For this review, use the dimensioned drawing (mm, ordinates from the lowest corner) and the shaded views. A direction names the side the tool comes from. Coordinates: 2 decimals unless noted, no trailing zeros. Loops run counter-clockwise (first coordinate to the right, second up) from the corner with the lowest first, then second, coordinate; pieces in that order, holes last. Notation, with made-up numbers: (23, 86) - (66, 86) arc R21 ccw to (66, 101) - close; hole circle Ø11 at (73, 13). An arc over 180 degrees is marked (long way). Answer in a Markdown table with one row per item. Add a question column.
(1) We need section D-D, the plane x = 14. Write out the cut boundary in (y, z), plus the area to 3 significant figures.
(2) The part is to be moulded in two halves that separate along X. For the marked faces 4, 5, 6 and 7, say which applies: released by +X, released by -X, zero draft, split by the parting line, or undercut.
(3) To check wall thickness, follow L1, parallel to Y at x = 72.3, z = 0.8; L2, parallel to X at y = 2.5, z = 1.25; L3, parallel to X at y = 50.7, z = 1.05. State the ranges of each line that lie inside material, in increasing order. Write a range as [from, to].
(4) We need section B-B, the plane z = 3.75. Write out the cut boundary in (x, y).
(5) We need section A-A, the plane y = 50.7. Write out the cut boundary in (x, z), plus the area to 3 significant figures.
(6) We need section C-C, the plane x = 72.3. Write out the cut boundary in (y, z).
(7) Clearance check with flat-ended pins moving along their axes: pin 1 (2 mm diameter, centred on x = 49.5, y = 18.5, fed in from +Z); pin 2 (7 mm diameter, centred on x = 26, y = 6.5, fed in from +Z); pin 3 (2.5 mm diameter, centred on y = 4, z = 8, fed in from -X). State where each tip first meets the part, or that it passes through.
(8) For the marked faces 1, 2 and 3, list the 3-axis set-ups (+Z, -Z, +X, -X, +Y, -Y) from which the entire face can be reached by the end or side of a thin tool; tool diameter is ignored.
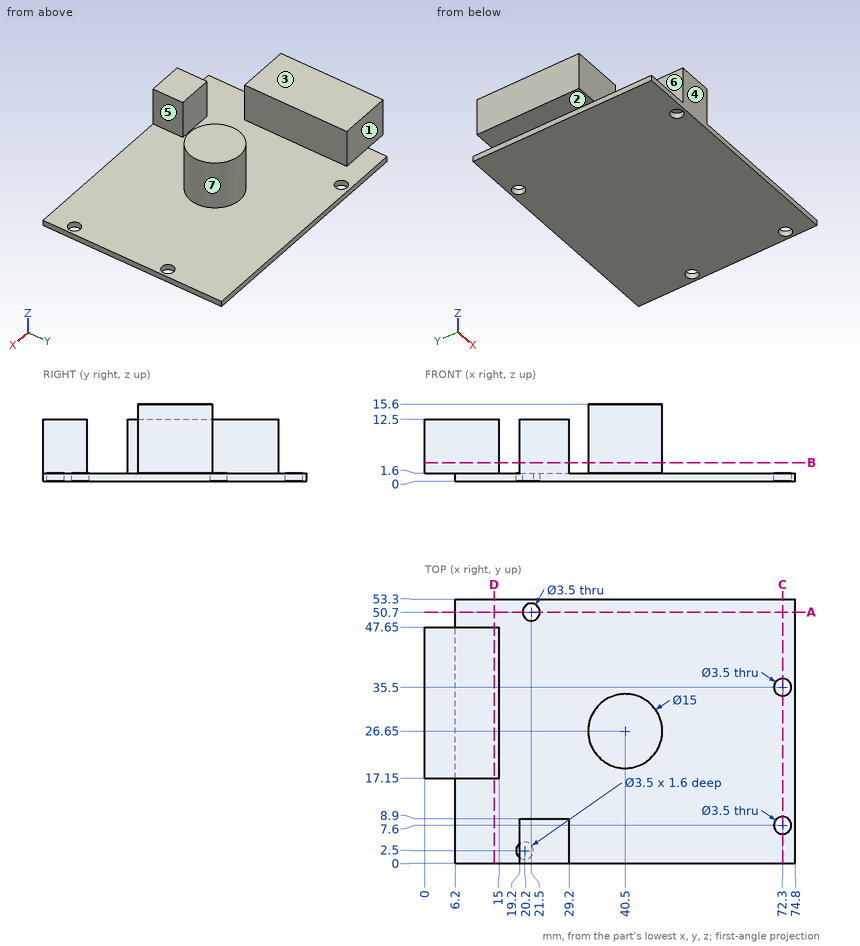
Responses:
| question | item | result |
|---|---|---|
| 1 | outline | (0, 0) - (53.3, 0) - (53.3, 1.6) - (47.65, 1.6) - (47.65, 12.5) - (17.15, 12.5) - (17.15, 1.6) - (0, 1.6) - close |
| 1 | area | 418 mm2 |
| 2 | face 4 | zero draft |
| 2 | face 5 | released by +X |
| 2 | face 6 | released by -X |
| 2 | face 7 | undercut |
| 3 | L1 | y = [0, 5.85], [9.35, 33.75], [37.25, 53.3] |
| 3 | L2 | x = [6.2, 18.45], [21.95, 74.8] |
| 3 | L3 | x = [6.2, 19.75], [23.25, 74.8] |
| 4 | outline | (0, 17.15) - (15, 17.15) - (15, 47.65) - (0, 47.65) - close; (19.2, 0) - (29.2, 0) - (29.2, 8.9) - (19.2, 8.9) - close; circle Ø15 at (40.5, 26.65) |
| 5 | outline | (6.2, 0) - (19.75, 0) - (19.75, 1.6) - (6.2, 1.6) - close; (23.25, 0) - (74.8, 0) - (74.8, 1.6) - (23.25, 1.6) - close |
| 5 | area | 104 mm2 |
| 6 | outline | (0, 0) - (5.85, 0) - (5.85, 1.6) - (0, 1.6) - close; (9.35, 0) - (33.75, 0) - (33.75, 1.6) - (9.35, 1.6) - close; (37.25, 0) - (53.3, 0) - (53.3, 1.6) - (37.25, 1.6) - close |
| 7 | pin 1 | stops at z = 1.6 |
| 7 | pin 2 | stops at z = 12.5 |
| 7 | pin 3 | stops at x = 19.2 |
| 8 | face 1 | +Z, +X, -X, +Y |
| 8 | face 2 | -Z, -X, +Y, -Y |
| 8 | face 3 | +Z, -X, +Y, -Y |
